Autodesk Inventor part; units mm, degrees
ref_plane "YZ Plane" through (0, 0, 0) normal (1, 0, 0) x (0, 1, 0)
ref_plane "XZ Plane" through (0, 0, 0) normal (0, 1, 0) x (-1, 0, 0)
ref_plane "XY Plane" through (0, 0, 0) normal (0, 0, 1) x (1, 0, 0)
sketch "Sketch1" plane through (0, 0, 0) normal (0, 0, 1) x (1, 0, 0)
  line L0 (0, 0) -> (0, 40.5449) construction
  line L1 (0, 0) -> (42.3786, 0) construction
  line L2 (-57.15, 76.2) -> (57.15, 76.2)
  line L3 (57.15, 76.2) -> (57.15, -76.2)
  line L4 (57.15, -76.2) -> (-57.15, -76.2)
  line L5 (-57.15, -76.2) -> (-57.15, 76.2)
  dimension "d0" = 152.4
  dimension "d1" = 114.3
extrude "Extrusion1" add sketch "Sketch1" along normal blind 3.175
sketch "Sketch2" plane through (0, 0, 3.175) normal (0, 0, 1) x (1, 0, 0)
  line L0 (57.15, 76.2) -> (-57.15, 76.2)
  line L1 (-57.15, 76.2) -> (-57.15, -76.2)
  point P0 (0, 0)
  point P1 (0, 38.1)
  dimension "d4" = 38.1
  dimension "d5" = 57.15
hole "Hole1" at (0, 38.1, 3.175) direction (0, 0, -1) diameter 12.7 end through all
sketch "Sketch3" plane through (0, 0, 3.175) normal (0, 0, 1) x (1, 0, 0)
  line L0 (-57.15, -76.2) -> (57.15, -76.2)
  line L1 (-57.15, 76.2) -> (-57.15, -76.2)
  point P0 (0, 0)
  point P1 (-50.8, -69.85)
  dimension "d13" = 6.35
  dimension "d14" = 6.35
hole "Hole2" at (-50.8, -69.85, 3.175) direction (0, 0, -1) diameter 3.175 end through all
mirror "Mirror1" about plane through (0, 0, 0) normal (1, 0, 0) of "Hole2"
mirror "Mirror2" about plane through (0, 0, 0) normal (0, 1, 0) of "Hole2", "Mirror1"
sketch "Sketch4" plane through (0, 0, 3.175) normal (0, 0, 1) x (1, 0, 0)
  line L0 (-57.15, -76.2) -> (57.15, -76.2)
  line L1 (-57.15, 76.2) -> (-57.15, -76.2)
  point P0 (0, 0)
  point P1 (0, -57.15)
  dimension "d22" = 19.05
  dimension "d23" = 57.15
hole "Hole3" at (0, -57.15, 3.175) direction (0, 0, -1) diameter 12.7 end through all
properties part number "GearBoxRearPlate"
Input: part model. Units: mm. Frame: model coordinates. Give positions to 0.01 mm unless a question says otherwise; leave off trailing zeros. Loops run counter-clockwise (first coordinate to the right, second up) from the corner with the lowest first, then second, coordinate; pieces in that order, holes last. Notation, with made-up numbers: M -25.75,-11.75 L 25.25,-11.75 A24 cw 25.25,16.25 Z; hole C 59.25,68.25 d11. An arc over 180 degrees is marked long. Use one line per item in the form item = value.
1. First-contact query: pin 1 (1.9 mm diameter, centred on x = -50.8, y = 69.85, fed in from -Z) (3 decimals). Flat tip, straight axial feed; report the tip coordinate or a pass-through.
Numbers:
pin_1 = through
2. Line query: L1, parallel to Y at x = -50.8, z = 1.35; L2, parallel to X at y = 69.85, z = 1.25; L3, parallel to Y at x = 50, z = 2.1. Output: solid intervals per line, ascending.
Numbers:
L1 = -76.2 to -71.44, -68.26 to 68.26, 71.44 to 76.2
L2 = -57.15 to -52.39, -49.21 to 49.21, 52.39 to 57.15
L3 = -76.2 to -71.22, -68.48 to 68.48, 71.22 to 76.2
3. Section query A-A, the plane y = 69.85. Count the separate pieces of the cut face and the enclosed holes in it, and give its area (3 significant figures).
Numbers:
separate_pieces = 3
enclosed_holes = 0
area = 343 mm²
4. Section query D-D, the plane y = 38.1. Return the cut outline in (x, z) (3 decimals), and give its area (3 significant figures).
Numbers:
outline = M -57.15,0 L -6.35,0 L -6.35,3.175 L -57.15,3.175 Z; M 6.35,0 L 57.15,0 L 57.15,3.175 L 6.35,3.175 Z
area = 323 mm²
5. Section query B-B, the plane x = 50.8. Return the cut outline in (y, z) (1 decimal).
Numbers:
outline = M -76.2,0 L -71.4,0 L -71.4,3.2 L -76.2,3.2 Z; M -68.3,0 L 68.3,0 L 68.3,3.2 L -68.3,3.2 Z; M 71.4,0 L 76.2,0 L 76.2,3.2 L 71.4,3.2 Z
6. Pull-direction query (X, two-part tool) for faces 1 (the face through (51.873, 68.68, 1.565)), 2 (the face through (57.15, 1, 2)), 3 (the face through (-1, 1, 3.175)); classes: released by +X, released by -X, zero draft, split by the parting line, or undercut.
Numbers:
face_1 = undercut
face_2 = released by +X
face_3 = zero draft
